Model file for the job. Use its own axes, mm. Give positions to 0.01 mm unless a question says otherwise; leave off trailing zeros. Order: outer loops, then holes, each group sorted by start corner. A loop starts at its lowest first (then second) coordinate and runs counter-clockwise, first axis right, second up. Notation, with made-up numbers: M -16,6 L -7,6 A25 cw -7,34 Z; hole C 71,74.25 d9. An arc over 180 degrees is marked long. Return JSON: item names as keys, results as strings. Group by question number.
1. Slice it at D-D on x = 9. List the corners of the cut face in (y, z).
2. Slice it at B-B on z = 0. List the corners of the cut face in (x, y).
3. Wall check: probe 1 along Z at (x, y) = (0, -0.5); probe 2 along Z at (x, y) = (80, 0.15); probe 3 along X at (y, z) = (1.45, 0.25). Give the ranges that are in metal, low to high. Write a range as [from, to].
4. Pin check, flat tip, straight feed: pin 1 (1 mm diameter, centred on x = 68, y = -1, fed in from +Z). Stop position of the tip, or through.
5. Slice it at C-C on y = -0.9. List the corners of the cut face in (x, z).
6. Slice it at A-A on x = 80. List the corners of the cut face in (y, z), then the cut area to 3 significant figures.
Autodesk Inventor part; units mm, degrees
ref_plane "YZ Plane" through (0, 0, 0) normal (1, 0, 0) x (0, 1, 0)
ref_plane "XZ Plane" through (0, 0, 0) normal (0, 1, 0) x (-1, 0, 0)
ref_plane "XY Plane" through (0, 0, 0) normal (0, 0, 1) x (1, 0, 0)
sketch "草圖1" plane through (0, 0, 0) normal (0, 1, 0) x (-1, 0, 0)
  circle A0 centre (0, 0) radius 1.5
  circle A1 centre (0, 0) radius 4
  line L0 (0, 0) -> (-80, 0)
  circle A2 centre (-80, 0) radius 1.5
  arc A3 (-76.9095, 5.1429) -> (-76.9095, -5.1429) centre (-80, 0) ccw
  line L1 (0, 4) -> (-72.7889, 4)
  line L2 (0, -4) -> (-72.7889, -4)
  arc A4 (-76.9095, 5.1429) -> (-72.7889, 4) centre (-72.7889, 12) ccw
  arc A5 (-72.7889, -4) -> (-76.9095, -5.1429) centre (-72.7889, -12) ccw
  point P0 (-75.5279, 4)
  point P1 (-75.5279, -4)
  dimension "d0" = 3
  dimension "d1" = 8
  dimension "d2" = 80
  dimension "d3" = 3
  dimension "d4" = 12
  dimension "d5" = 8
extrude "擠出1" add sketch "草圖1" along normal mid plane 3
properties part number "連接1"
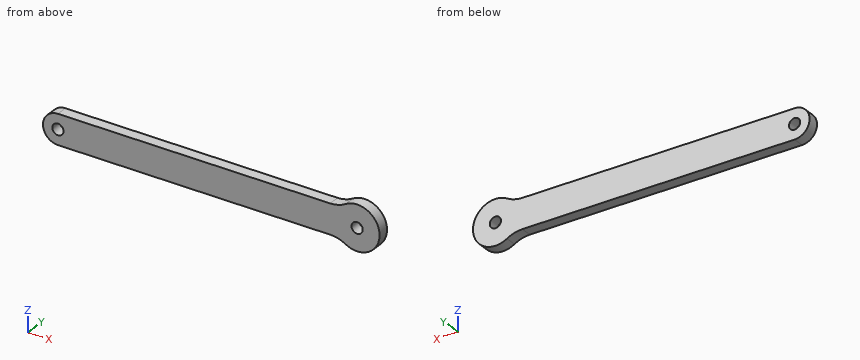
Result:
{
 "1": {"outline": "M -1.5,-4 L 1.5,-4 L 1.5,4 L -1.5,4 Z"},
 "2": {"outline": "M -4,-1.5 L -1.5,-1.5 L -1.5,1.5 L -4,1.5 Z; M 1.5,-1.5 L 78.5,-1.5 L 78.5,1.5 L 1.5,1.5 Z; M 81.5,-1.5 L 86,-1.5 L 86,1.5 L 81.5,1.5 Z"},
 "3": {"probe 1": "z = [-4, -1.5], [1.5, 4]", "probe 2": "z = [-6, -1.5], [1.5, 6]", "probe 3": "x = [-3.99, -1.48], [1.48, 78.52], [81.48, 85.99]"},
 "4": {"pin 1": "stops at z = 4"},
 "5": {"outline": "M 0,-4 L 72.79,-4 A8 cw 76.91,-5.14 A6 ccw long 76.91,5.14 A8 cw 72.79,4 L 0,4 A4 ccw Z; hole C 0,0 d3; hole C 80,0 d3"},
 "6": {"outline": "M -1.5,-6 L 1.5,-6 L 1.5,-1.5 L -1.5,-1.5 Z; M -1.5,1.5 L 1.5,1.5 L 1.5,6 L -1.5,6 Z", "area": "27.0 mm2"}
}
